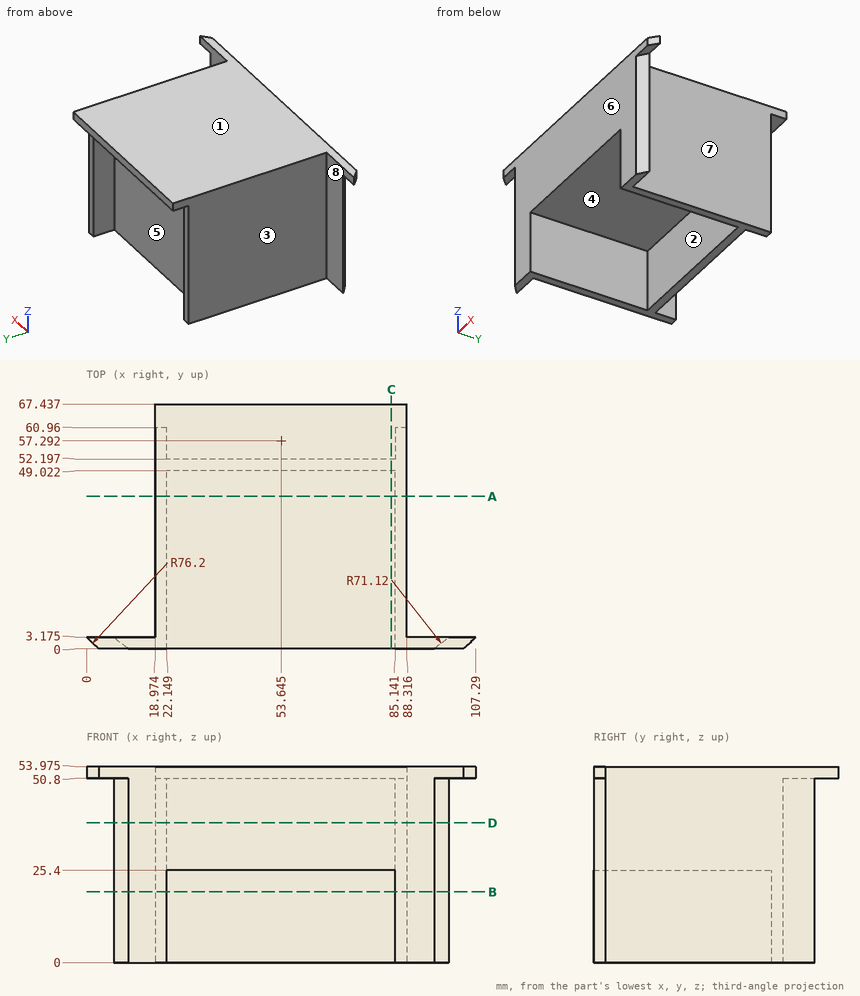
Geometry: see drawing. Coordinates: mm, zero at the bounding-box minimum. A direction names the side the tool comes from. Coordinates: 2 decimals unless noted, no trailing zeros. Order: outer loops, then holes, each group sorted by start corner. A loop starts at its lowest first (then second) coordinate and runs counter-clockwise, first axis right, second up. Notation, with made-up numbers: M 55,-34 L 90,-34 A24 cw 90,-4 Z; hole C 76,-35 d10. An arc over 180 degrees is marked long. Write item = value, one per line. Start each with the question number.
(1) Section B-B on z = 19.5. Output: boundary loops of the cut face in (x, y) (1 decimal).
(2) Reachability of the marked faces 4, 5, 6, 7 and 8 from +Z, -Z, +X, -X, +Y, -Y: full face, straight path, thin tool, end or side. Return the list, or none.
(3) Section C-C on x = 84. Output: boundary loops of the cut face in (y, z) (1 decimal).
(4) First-contact query: P1, Ø15, axis at x = 6, z = 21, coming from the +Y side (3 decimals); P2, Ø1, axis at x = 99.5, y = 1, coming from the -Z side; P3, Ø3, axis at x = 18, z = 16, coming from the +Y side. Flat tips, straight axial feed; report the tip coordinate or a pass-through.
(5) Pull-direction query (X, two-part tool) for the marked faces 1, 2 and 3; classes: released by +X, released by -X, zero draft, split by the parting line, or undercut.
(6) Section D-D on z = 38.5. Output: boundary loops of the cut face in (x, y) (1 decimal), and give its area (3 significant figures).
(7) Line query: line 1 along X through (y, z) = (14, 8.5); line 2 along Y through (x, z) = (66.5, 3); line 3 along Z through (x, y) = (64.5, 15) (1 decimal). Output: solid intervals per line, ascending. Write a range as [from, to].
(8) Section A-A on y = 42. Output: boundary loops of the cut face in (x, z) (1 decimal), and give its area (3 significant figures).
Result set:
q1.outline = M 7.5,3.2 A71.1 ccw 11.5,0 L 22.1,0 L 22.1,49 L 85.1,49 L 85.1,0 L 95.8,0 A71.1 ccw 99.8,3.2 L 88.3,3.2 L 88.3,61 L 85.1,61 L 85.1,52.2 L 22.1,52.2 L 22.1,61 L 19,61 L 19,3.2 Z
q2.face_4 = -Z, -Y
q2.face_5 = -Z, +Y
q2.face_6 = +Z, -Z, +X, -X, -Y
q2.face_7 = +Z, -Z, +X, +Y
q2.face_8 = +Z, -Z, -X, +Y
q3.outline = M 0,25.4 L 49,25.4 L 49,0 L 52.2,0 L 52.2,50.8 L 67.4,50.8 L 67.4,54 L 0,54 Z
q4.P1 = 3.175
q4.P2 = 50.8
q4.P3 = 60.96
q5.face_1 = zero draft
q5.face_2 = undercut
q5.face_3 = released by -X
q6.outline = M 7.5,3.2 A71.1 ccw 11.5,0 L 95.8,0 A71.1 ccw 99.8,3.2 L 88.3,3.2 L 88.3,61 L 85.1,61 L 85.1,52.2 L 22.1,52.2 L 22.1,61 L 19,61 L 19,3.2 Z
q6.area = 3,740 mm²
q7.line_1 = [18.97, 22.15], [85.14, 88.32]
q7.line_2 = [49.02, 52.2]
q7.line_3 = [25.4, 54]
q8.outline = M 19,0 L 22.1,0 L 22.1,25.4 L 85.1,25.4 L 85.1,0 L 88.3,0 L 88.3,54 L 19,54 Z
q8.area = 2,140 mm²
